Verification items for the finished model (mm, model axes). A direction names the side the tool comes from. Round coordinates to 2 decimals unless told otherwise and drop trailing zeros. Write each loop counter-clockwise with the first axis right and the second up, starting at its lowest first coordinate (ties: lowest second). Pieces come first, ordered by that corner, then holes. Notation, with made-up numbers: (-34, 86) - (-14, 86) arc R29 cw to (-14, 107) - close; hole circle Ø6 at (49, 40). An arc over 180 degrees is marked (long way). Answer as a JSON object with one key per item and string values. Group by question number.
1) Section check C-C (z = -39). Enter the section's corners in (x, y).
2) Section check B-B (z = -17.5). Enter the section's corners in (x, y).
3) Section check A-A (x = 25). Enter the section's corners in (y, z), then the cut area to 3 significant figures.
4) Set-up check for faces 1 (the cylindrical face through (17.78, 2.54, -5.77)), 2 (the cylindrical face through (53.99, 2.83, -27.48)), 3 (the cylindrical face through (23.5, 2.57, 1.48)), 4 (the cylindrical face through (-3.99, 2.83, -27.48)): record each of +Z, -Z, +X, -X, +Y, -Y from which the full face is reachable in a straight line by a thin tool's end or side.
5) Section check D-D (z = -11). Enter the section's corners in (x, y).
6) Mould release check, pull along Z, two halves, no side actions. Record for faces 5 (the cylindrical face through (-1.48, 2.57, -23.5)), 6 (the flat face through (55, 3, -25)), 7 (the cylindrical face through (38.45, 2.46, -23.71)): +Z half, -Z half, draft (parallel to the pull), parting line (faces both ways), or undercut.
7) Go/stop test with flat-tipped pins: pin 1 Ø4.5 at (x, z) = (12.74, -25) entering from -Y; pin 2 Ø1.5 at (x, y) = (8.5, 0.5) entering from -Z; pin 3 Ø1.5 at (x, z) = (31, -17.5) entering from -Y; pin 4 Ø1.5 at (y, z) = (2.5, -29) entering from +X. Record where each tip stops, or that it passes through.
8) Thickness scan on line 1 (X direction, y = 1.1, z = -25); line 2 (X direction, y = 3.65, z = -11); line 3 (X direction, y = 1.25, z = -39). Record the ranges inside material, lowest first.
```python
from build123d import *

# Parameters (mm, degrees)
SKETCH_1_W          = 50
SKETCH_1_H          = 50
EXTRUDE_1_DEPTH     = 5
SKETCH_2_R          = 3
CUT_EXTRUDE_1_DEPTH = 71.887234394
SKETCH_3_R          = 1.25
CUT_EXTRUDE_2_DEPTH = 71.887234394
SKETCH_8_R          = 1.75
CUT_EXTRUDE_4_DEPTH = 71.887234394
SKETCH_9_R          = 2.5
EXTRUDE_2_DEPTH     = 5
SKETCH_10_R         = 2.5
SKETCH_10_R_2       = 1.5
CUT_EXTRUDE_5_DEPTH = 3
SKETCH_11_R         = 2.5
EXTRUDE_3_DEPTH     = 5
SKETCH_12_R         = 2.5
SKETCH_12_R_2       = 1.5
CUT_EXTRUDE_7_DEPTH = 3


with BuildPart() as part:
    # 草图1 → 凸台-拉伸1 (new body)
    with BuildSketch(Plane(origin=(0, 0, 0), x_dir=(1, 0, 0), z_dir=(0, 1, 0))):
        with Locations((25, 25)):
            Rectangle(SKETCH_1_W, SKETCH_1_H)
    extrude(amount=EXTRUDE_1_DEPTH)

    # 草图2 → 切除-拉伸1 (cut, through all)
    with BuildSketch(Plane(origin=(0, 5, 0), x_dir=(1, 0, 0), z_dir=(0, 1, 0))):
        with Locations(Location((25, 39, 0), (0, 0, 270))):
            Circle(SKETCH_2_R)
        with Locations(Location((11, 11, 0), (0, 0, 270))):
            Circle(SKETCH_2_R)
        with Locations(Location((39, 11, 0), (0, 0, 270))):
            Circle(SKETCH_2_R)
    extrude(amount=-CUT_EXTRUDE_1_DEPTH, mode=Mode.SUBTRACT)

    # 草图3 → 切除-拉伸2 (cut, through all)
    with BuildSketch(Plane(origin=(0, 5, 0), x_dir=(1, 0, 0), z_dir=(0, 1, 0))):
        with Locations(Location((19, 17.5, 0), (0, 0, 270))):
            Circle(SKETCH_3_R)
        with Locations(Location((31, 17.5, 0), (0, 0, 270))):
            Circle(SKETCH_3_R)
        with Locations(Location((19, 5.5, 0), (0, 0, 270))):
            Circle(SKETCH_3_R)
        with Locations(Location((31, 5.5, 0), (0, 0, 270))):
            Circle(SKETCH_3_R)
    extrude(amount=-CUT_EXTRUDE_2_DEPTH, mode=Mode.SUBTRACT)

    # 草图8 → 切除-拉伸4 (cut, through all)
    with BuildSketch(Plane.XZ):
        with Locations(Location((46.372516673, -22, 0), (0, 0, 270))):
            Circle(SKETCH_8_R)
        with Locations(Location((46.372516673, -28, 0), (0, 0, 270))):
            Circle(SKETCH_8_R)
        with Locations(Location((37.264513071, -25, 0), (0, 0, 270))):
            Circle(SKETCH_8_R)
        with Locations(Location((12.735486929, -25, 0), (0, 0, 270))):
            Circle(SKETCH_8_R)
        with Locations(Location((3.627483327, -28, 0), (0, 0, 270))):
            Circle(SKETCH_8_R)
        with Locations(Location((3.627483327, -22, 0), (0, 0, 270))):
            Circle(SKETCH_8_R)
    extrude(amount=-CUT_EXTRUDE_4_DEPTH, mode=Mode.SUBTRACT)

    # 草图9 → 凸台-拉伸2 (add)
    with BuildSketch(Plane.XY):
        with Locations(Location((25, 2.5, 0), (0, 0, 270))):
            Circle(SKETCH_9_R)
    extrude_2 = extrude(amount=EXTRUDE_2_DEPTH)

    # 草图10 → 切除-拉伸5 (cut)
    with BuildSketch(Plane.XY):
        with Locations((25, 2.5)):
            Circle(SKETCH_10_R)
        with Locations((25, 2.5)):
            Circle(SKETCH_10_R_2, mode=Mode.SUBTRACT)
    cut_extrude_5 = extrude(amount=CUT_EXTRUDE_5_DEPTH, mode=Mode.SUBTRACT)

    # 草图11 → 凸台-拉伸3 (add)
    with BuildSketch(Plane(origin=(50, 0, 0), x_dir=(0, 0, -1), z_dir=(1, 0, 0))):
        with Locations(Location((25, 2.5, 0), (0, 0, 270))):
            Circle(SKETCH_11_R)
    extrude_3 = extrude(amount=EXTRUDE_3_DEPTH)

    # 草图12 → 切除-拉伸7 (cut)
    with BuildSketch(Plane(origin=(50, 0, 0), x_dir=(0, 0, -1), z_dir=(1, 0, 0))):
        with Locations((25, 2.5)):
            Circle(SKETCH_12_R)
        with Locations((25, 2.5)):
            Circle(SKETCH_12_R_2, mode=Mode.SUBTRACT)
    cut_extrude_7 = extrude(amount=CUT_EXTRUDE_7_DEPTH, mode=Mode.SUBTRACT)

    # 镜向1: 凸台-拉伸3, 切除-拉伸7 across plane
    add(extrude_3.mirror(Plane.ZY.offset(-25)))
    add(cut_extrude_7.mirror(Plane.ZY.offset(-25)), mode=Mode.SUBTRACT)

    # 镜向2: 凸台-拉伸2, 切除-拉伸5 across plane
    add(extrude_2.mirror(Plane(origin=(0, 0, -25), x_dir=(1, 0, 0), z_dir=(0, 0, -1))))
    add(cut_extrude_5.mirror(Plane(origin=(0, 0, -25), x_dir=(1, 0, 0), z_dir=(0, 0, -1))), mode=Mode.SUBTRACT)


solid = part.part
```
Returned:
{
 "1": {"outline": "(0, 0) - (22, 0) - (22, 5) - (0, 5) - close; (28, 0) - (50, 0) - (50, 5) - (28, 5) - close"},
 "2": {"outline": "(0, 0) - (17.75, 0) - (17.75, 5) - (0, 5) - close; (20.25, 0) - (29.75, 0) - (29.75, 5) - (20.25, 5) - close; (32.25, 0) - (50, 0) - (50, 5) - (32.25, 5) - close"},
 "3": {"outline": "(0, -55) - (5, -55) - (5, -53) - (4, -53) - (4, -50) - (5, -50) - (5, -42) - (0, -42) - (0, -50) - (1, -50) - (1, -53) - (0, -53) - close; (0, -36) - (5, -36) - (5, 0) - (4, 0) - (4, 3) - (5, 3) - (5, 5) - (0, 5) - (0, 3) - (1, 3) - (1, 0) - (0, 0) - close", "area": "258 mm2"},
 "4": {"face 1": "+Y, -Y", "face 2": "+X", "face 3": "none", "face 4": "-X"},
 "5": {"outline": "(0, 0) - (8, 0) - (8, 5) - (0, 5) - close; (14, 0) - (36, 0) - (36, 5) - (14, 5) - close; (42, 0) - (50, 0) - (50, 5) - (42, 5) - close"},
 "6": {"face 5": "parting line", "face 6": "draft", "face 7": "undercut"},
 "7": {"pin 1": "y = 0", "pin 2": "z = -50", "pin 3": "through", "pin 4": "x = 50"},
 "8": {"line 1": "-5 to 10.99, 14.49 to 35.51, 39.01 to 55", "line 2": "0 to 8, 14 to 36, 42 to 50", "line 3": "0 to 22, 28 to 50"}
}
